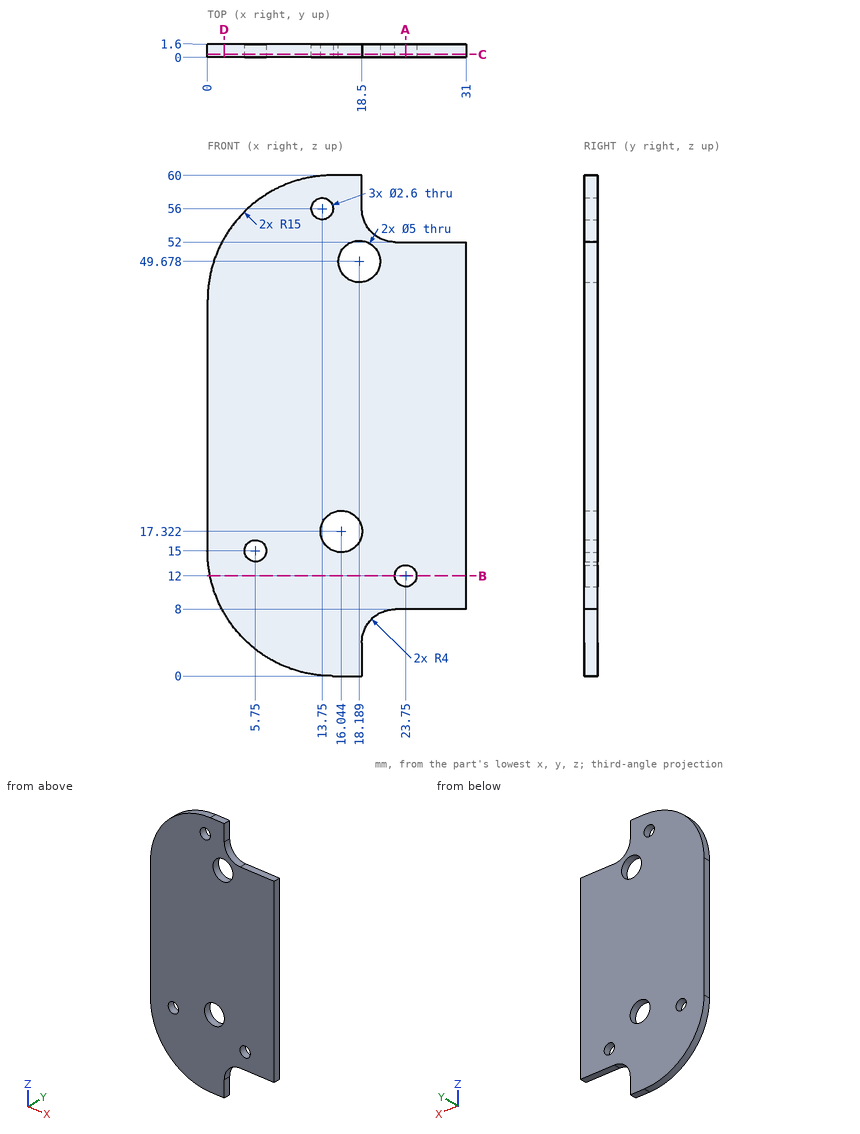
Design review of the part shown in the three views and the two pictorial views. Dimensions are in mm from the part's minimum x, y and z. Give positions to 0.01 mm unless a question says otherwise; leave off trailing zeros. Loops run counter-clockwise (first coordinate to the right, second up) from the corner with the lowest first, then second, coordinate; pieces in that order, holes last. Notation, with made-up numbers: (39.25, 22) -> (50.25, 22) arc R11 cw to (50.25, 35) -> close; hole circle Ø11 at (26.5, 24.25). An arc over 180 degrees is marked (long way). One line per question, with ' | ' between items.
1) To check wall thickness, follow probe 1 along Z at (x, y) = (13.75, 1.2); probe 2 along Z at (x, y) = (17, 0.1); probe 3 along Z at (x, y) = (5.75, 0.6). State the ranges of each line that lie inside material, in increasing order.
Resolved:
probe 1: z = 0.05 to 16.33, 18.32 to 54.7, 57.3 to 59.95 | probe 2: z = 0 to 15.01, 19.63 to 47.48, 51.88 to 60 | probe 3: z = 3.19 to 13.7, 16.3 to 56.81
2) We need section B-B (z = 12). Write out the cut boundary in (x, y), plus the area to 3 significant figures.
Resolved:
outline: (0.3, 0) -> (22.45, 0) -> (22.45, 1.6) -> (0.3, 1.6) -> close; (25.05, 0) -> (31, 0) -> (31, 1.6) -> (25.05, 1.6) -> close | area: 45.0 mm2
3) Insertion check: pin 1 Ø0.5 at (y, z) = (1, 2.5) entering from +X; pin 2 Ø0.5 at (x, y) = (26.5, 0.5) entering from -Z; pin 3 Ø0.8 at (x, y) = (27.5, 1) entering from +Z. Each pin has a flat end and moves straight along its axis. Give the tip position at first contact, or say it passes through.
Resolved:
pin 1: stops at x = 18.5 | pin 2: stops at z = 8 | pin 3: stops at z = 52
4) We need section A-A (x = 23.75). Write out the cut boundary in (y, z), plus the area to 3 significant figures.
Resolved:
outline: (0, 8) -> (1.6, 8) -> (1.6, 10.7) -> (0, 10.7) -> close; (0, 13.3) -> (1.6, 13.3) -> (1.6, 52) -> (0, 52) -> close | area: 66.2 mm2
5) We need section D-D (x = 2). Write out the cut boundary in (y, z).
Resolved:
outline: (0, 7.52) -> (1.6, 7.52) -> (1.6, 52.48) -> (0, 52.48) -> close
6) We need section C-C (y = 0.35). Write out the cut boundary in (x, z), plus the area to 3 significant figures.
Resolved:
outline: (0, 15) arc R15 ccw to (15, 0) -> (18.5, 0) -> (18.5, 4) arc R4 cw to (22.5, 8) -> (31, 8) -> (31, 52) -> (22.5, 52) arc R4 cw to (18.5, 56) -> (18.5, 60) -> (15, 60) arc R15 ccw to (0, 45) -> close; hole circle Ø2.6 at (5.75, 15); hole circle Ø2.6 at (13.75, 56); hole circle Ø5 at (16.04, 17.32); hole circle Ø5 at (18.19, 49.68); hole circle Ø2.6 at (23.75, 12) | area: 1,520 mm2
